Geometry: final body of the model. Coordinates: model frame, mm. Give positions to 0.01 mm unless a question says otherwise; leave off trailing zeros. Loops run counter-clockwise (first coordinate to the right, second up) from the corner with the lowest first, then second, coordinate; pieces in that order, holes last. Notation, with made-up numbers: (11, 31) -> (26, 31) arc R26 ccw to (26, 55) -> close; hole circle Ø10 at (5, 21). An arc over 180 degrees is marked (long way). Answer in a Markdown table with one row per item. Add a question column.
1) Section query C-C (z = 3.75). Return the cut outline in (x, y).
2) Line query: line 1 (Y direction, x = 0, z = 4.9); line 2 (Z direction, x = 1, y = -0.25); line 3 (X direction, y = 2, z = 1.5). Output: solid intervals per line, ascending. Write a range as from..to.
3) Section query D-D (z = 1). Return the cut outline in (x, y).
4) Section query A-A (y = 0). Return the cut outline in (x, z).
5) Draft query along Y for faces 1 (the cylindrical face through (-1.08, -4.88, 3.16)), 2 (the flat face through (0, 0, 3)), 3 (the flat face through (0, 0, 0)), 4 (the cylindrical face through (0, -2, 5)). Return one class per face: +Y half, -Y half, draft (parallel to the pull), parting line (faces both ways), or undercut.
6) First-contact query: P1, Ø1.5, axis at x = -2.5, z = 4, coming from the -Y side; P2, Ø3, axis at y = 2.5, z = 1, coming from the +X side; P3, Ø0.9, axis at x = 0.5, y = -0.5, coming from the +Z side. Flat tips, straight axial feed; report the tip coordinate or a pass-through.
```python
from build123d import *

# Parameters (mm, degrees)
SCHIZZO1_R                   = 5
ESTRUSIONE_ESTRUSIONE1_DEPTH = 6
SCHIZZO2_R                   = 2
TAGLIO_ESTRUSIONE1_DEPTH     = 3
RACCORDO1_R                  = 0.5
RACCORDO2_R                  = 0.1


with BuildPart() as part:
    # Schizzo1 → Estrusione-Estrusione1 (new body)
    with BuildSketch(Plane.XY):
        Circle(SCHIZZO1_R)
    extrude(amount=ESTRUSIONE_ESTRUSIONE1_DEPTH)

    # Schizzo2 → Taglio-Estrusione1 (cut)
    with BuildSketch(Plane.XY.offset(6)):
        Circle(SCHIZZO2_R)
    extrude(amount=-TAGLIO_ESTRUSIONE1_DEPTH, mode=Mode.SUBTRACT)

    # Raccordo1
    raccordo1_edges = [part.edges().sort_by_distance(p)[0] for p in [
        (-5, 0, 0),
        (-2, 0, 3),
        (-2, 0, 6),
    ]]
    fillet(raccordo1_edges, radius=RACCORDO1_R)

    # Raccordo2
    raccordo2_edges = [part.edges().sort_by_distance(p)[0] for p in [
        (-5, 0, 6),
    ]]
    fillet(raccordo2_edges, radius=RACCORDO2_R)


solid = part.part
```
Evaluation:
| question | item | result |
|---|---|---|
| 1 | outline | circle Ø10 at (0, 0); hole circle Ø4 at (0, 0) |
| 2 | line 1 | -5..-2, 2..5 |
| 2 | line 2 | 0..3 |
| 2 | line 3 | -4.58..4.58 |
| 3 | outline | circle Ø10 at (0, 0) |
| 4 | outline | (-5, 0.5) arc R0.5 ccw to (-4.5, 0) -> (4.5, 0) arc R0.5 ccw to (5, 0.5) -> (5, 5.9) arc R0.1 ccw to (4.9, 6) -> (2.5, 6) arc R0.5 ccw to (2, 5.5) -> (2, 3.5) arc R0.5 cw to (1.5, 3) -> (-1.5, 3) arc R0.5 cw to (-2, 3.5) -> (-2, 5.5) arc R0.5 ccw to (-2.5, 6) -> (-4.9, 6) arc R0.1 ccw to (-5, 5.9) -> close |
| 5 | face 1 | parting line |
| 5 | face 2 | undercut |
| 5 | face 3 | draft |
| 5 | face 4 | undercut |
| 6 | P1 | y = -4.68 |
| 6 | P2 | x = 4.9 |
| 6 | P3 | z = 3 |
